Answer from the drawing. Dimensions are ordinates in mm from the lowest x, y and z of the part. A direction names the side the tool comes from. Coordinates: 2 decimals unless noted, no trailing zeros. Write each loop counter-clockwise with the first axis right and the second up, starting at its lowest first coordinate (ties: lowest second). Pieces come first, ordered by that corner, then holes. Notation, with made-up numbers: (30.25, 75.5) -> (35.25, 75.5) arc R23 ccw to (35.25, 100.5) -> close; hole circle Ø6 at (3.5, 38). An arc over 180 degrees is marked (long way). Return JSON: item names as keys, results as strings.
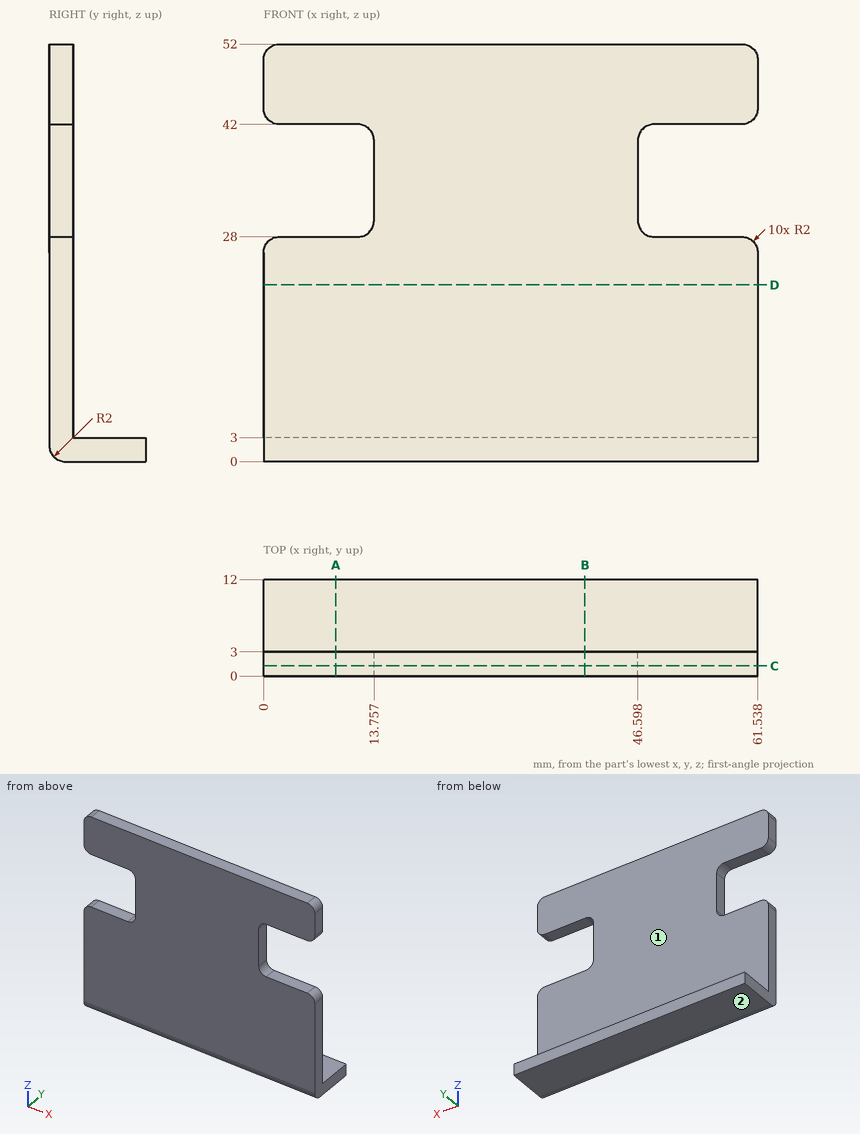
1. Consider L1, parallel to Z at x = 54, y = 2.5; L2, parallel to Z at x = 7, y = 10.25; L3, parallel to X at y = 1.75, z = 33.5. Determine where each line is inside the solid, lowest interval first.
Taken from the geometry:
{"L1": "z = 0 to 28, 42 to 52", "L2": "z = 0 to 3", "L3": "x = 13.76 to 46.6"}
2. A tool of negligible diameter and unlimited length cuts with its end or side. For the marked faces 1 and 2, from which of +Z, -Z, +X, -X, +Y, -Y can it reach the whole face along a straight path? Write none if from no direction.
Taken from the geometry:
{"face 1": "+Z, +X, -X, +Y", "face 2": "-Z, +X, -X, +Y, -Y"}
3. The part is cut by section C-C (y = 1.25). Determine the outline of the cut face in (x, z).
Taken from the geometry:
{"outline": "(0, 0.15) -> (61.54, 0.15) -> (61.54, 26) arc R2 ccw to (59.54, 28) -> (48.6, 28) arc R2 cw to (46.6, 30) -> (46.6, 40) arc R2 cw to (48.6, 42) -> (59.54, 42) arc R2 ccw to (61.54, 44) -> (61.54, 50) arc R2 ccw to (59.54, 52) -> (2, 52) arc R2 ccw to (0, 50) -> (0, 44) arc R2 ccw to (2, 42) -> (11.76, 42) arc R2 cw to (13.76, 40) -> (13.76, 30) arc R2 cw to (11.76, 28) -> (2, 28) arc R2 ccw to (0, 26) -> close"}
4. The part is cut by section A-A (x = 9). Determine the outline of the cut face in (y, z), then the cut area to 3 significant figures.
Taken from the geometry:
{"outline": "(0, 2) arc R2 ccw to (2, 0) -> (12, 0) -> (12, 3) -> (3, 3) -> (3, 28) -> (0, 28) -> close; (0, 42) -> (3, 42) -> (3, 52) -> (0, 52) -> close", "area": "140 mm2"}
5. The part is cut by section D-D (z = 22). Determine the outline of the cut face in (x, y).
Taken from the geometry:
{"outline": "(0, 0) -> (61.54, 0) -> (61.54, 3) -> (0, 3) -> close"}
6. Flat-ended cylindrical pins translate along their axes: pin 1 Ø2.5 at (x, y) = (7, 1) entering from -Z; pin 2 Ø3 at (x, y) = (36.5, 10.5) entering from +Z; pin 3 Ø1.5 at (y, z) = (2, 37) entering from +X; pin 4 Ø24.5 at (x, z) = (22.5, 29) entering from +Y. Find the tip coordinate at first contact, or state that the pin passes through.
Taken from the geometry:
{"pin 1": "stops at z = 0", "pin 2": "stops at z = 3", "pin 3": "stops at x = 46.6", "pin 4": "stops at y = 3"}
7. The part is cut by section B-B (x = 40). Determine the outline of the cut face in (y, z), then the cut area to 3 significant figures.
Taken from the geometry:
{"outline": "(0, 2) arc R2 ccw to (2, 0) -> (12, 0) -> (12, 3) -> (3, 3) -> (3, 52) -> (0, 52) -> close", "area": "182 mm2"}
